Verification items for the finished model (mm, model axes). A direction names the side the tool comes from. Round coordinates to 2 decimals unless told otherwise and drop trailing zeros. Order: outer loops, then holes, each group sorted by start corner. A loop starts at its lowest first (then second) coordinate and runs counter-clockwise, first axis right, second up. Notation, with made-up numbers: (-13, 48.5) -> (23, 48.5) arc R22 ccw to (23, 66.5) -> close; hole circle Ø5 at (-30, 27). An arc over 180 degrees is marked (long way). Write item = value, one per line. Start each with the question number.
from build123d import *

# Parameters (mm, degrees)
BOSS_EXTRUDE1_DEPTH = 3
SKETCH2_R           = 1.5
CUT_EXTRUDE1_DEPTH  = 12


with BuildPart() as part:
    # Sketch1 → Boss-Extrude1 (new, symmetric)
    with BuildSketch(Plane.XY):
        with BuildLine():
            Line((-6.75, 20.40625), (6.75, 20.40625))
            ThreePointArc((6.75, 20.40625), (8.164213562, 19.820463562), (8.75, 18.40625))
            Line((8.75, 18.40625), (8.75, -7.09375))
            Line((8.75, -7.09375), (15.35, -7.09375))
            Line((15.35, -7.09375), (15.35, 26.40625))
            Line((15.35, 26.40625), (-15.35, 26.40625))
            Line((-15.35, 26.40625), (-15.35, -7.09375))
            Line((-15.35, -7.09375), (-8.75, -7.09375))
            Line((-8.75, -7.09375), (-8.75, 18.40625))
            ThreePointArc((-8.75, 18.40625), (-8.164213562, 19.820463562), (-6.75, 20.40625))
        make_face()
    extrude(amount=BOSS_EXTRUDE1_DEPTH, both=True)

    # Sketch2 → Cut-Extrude1 (cut)
    with BuildSketch(Plane.XZ.offset(7.09375)):
        with Locations((-12.05, 0)):
            Circle(SKETCH2_R)
        with Locations(Location((12.05, 0, 0), (0, 0, 180))):
            Circle(SKETCH2_R)
    extrude(amount=-CUT_EXTRUDE1_DEPTH, mode=Mode.SUBTRACT)


solid = part.part
(1) Cross-section at C-C (z = 0). Enter the section's corners in (x, y).
(2) Scan lines: line 1 along X through (y, z) = (16, 0.55); line 2 along Z through (x, y) = (-12.05, -3.75). Record each from-to range of solid material in increasing order. Write a range as from..to.
(3) Cross-section at B-B (y = 6). Enter the section's corners in (x, z).
(4) Set-up check for faces 4 (the flat face through (0, 20.406, 0)), 5 (the flat face through (0, 21, 3)), 6 (the flat face through (-12, 4.906, 0)): record each of +Z, -Z, +X, -X, +Y, -Y from which the full face is reachable in a straight line by a thin tool's end or side.
(5) Cross-section at A-A (y = 2.5). Enter the section's corners in (x, z).
(6) Cross-section at D-D (x = -12.05). Enter the section's corners in (y, z).
(7) Depth check by flat-ended pin: pin 1 (1.5 mm diameter, centred on x = -2, z = 0.5, fed in from -Y); pin 2 (2.5 mm diameter, centred on x = -12.05, z = 0, fed in from -Y). Enter the tip coordinate at first touch or a pass-through.
(8) Draft check along Z on faces 1 (the flat face through (0, 21, -3)), 2 (the flat face through (-14, -7.094, 0)), 3 (the cylindrical face through (-13.55, -1.18, 0.07)). Enter one of: +Z half, -Z half, draft (parallel to the pull), parting line (faces both ways), or undercut.
Outcome:
q1.outline = (-15.35, -7.09) -> (-13.55, -7.09) -> (-13.55, 4.91) -> (-10.55, 4.91) -> (-10.55, -7.09) -> (-8.75, -7.09) -> (-8.75, 18.41) arc R2 cw to (-6.75, 20.41) -> (6.75, 20.41) arc R2 cw to (8.75, 18.41) -> (8.75, -7.09) -> (10.55, -7.09) -> (10.55, 4.91) -> (13.55, 4.91) -> (13.55, -7.09) -> (15.35, -7.09) -> (15.35, 26.41) -> (-15.35, 26.41) -> close
q2.line_1 = -15.35..-8.75, 8.75..15.35
q2.line_2 = -3..-1.5, 1.5..3
q3.outline = (-15.35, -3) -> (-8.75, -3) -> (-8.75, 3) -> (-15.35, 3) -> close; (8.75, -3) -> (15.35, -3) -> (15.35, 3) -> (8.75, 3) -> close
q4.face_4 = +Z, -Z, -Y
q4.face_5 = +Z, +X, -X, +Y, -Y
q4.face_6 = -Y
q5.outline = (-15.35, -3) -> (-8.75, -3) -> (-8.75, 3) -> (-15.35, 3) -> close; (8.75, -3) -> (15.35, -3) -> (15.35, 3) -> (8.75, 3) -> close; hole circle Ø3 at (-12.05, 0); hole circle Ø3 at (12.05, 0)
q6.outline = (-7.09, -3) -> (26.41, -3) -> (26.41, 3) -> (-7.09, 3) -> (-7.09, 1.5) -> (4.91, 1.5) -> (4.91, -1.5) -> (-7.09, -1.5) -> close
q7.pin_1 = 20.41
q7.pin_2 = 4.91
q8.face_1 = -Z half
q8.face_2 = draft
q8.face_3 = undercut
